Geometry: final body of the model. Coordinates: model frame, mm. Face numbers are marked on the shaded views. A direction names the side the tool comes from. Give positions to 0.01 mm unless a question says otherwise; leave off trailing zeros. Order: outer loops, then holes, each group sorted by start corner. A loop starts at its lowest first (then second) coordinate and runs counter-clockwise, first axis right, second up. Notation, with made-up numbers: (37.25, 64.5) - (67.25, 64.5) arc R34 ccw to (67.25, 96.5) - close; hole circle Ø9 at (71, 36.5). An arc over 180 degrees is marked (long way). Use one line per item in the form item = value.
from build123d import *

# Parameters (mm, degrees)
SKETCH1_W           = 39.99992
SKETCH1_H           = 19.99996
BOSS_EXTRUDE1_DEPTH = 9.0000074
BOSS_EXTRUDE2_DEPTH = 2.00000108
CHAMFER2_SIZE       = 1.00000054
SKETCH3_R           = 6.9999987
BOSS_EXTRUDE3_DEPTH = 1.00000054
SKETCH4_R           = 5.5000017
BOSS_EXTRUDE4_DEPTH = 1.00000054
SKETCH5_R           = 2.999994
CUT_EXTRUDE1_DEPTH  = 2.54
BOSS_EXTRUDE5_DEPTH = 1.999996
FILLET1_R           = 0.7500112
BOSS_EXTRUDE6_DEPTH = 0.50000027


with BuildPart() as part:
    # Sketch1 → Boss-Extrude1 (new body)
    with BuildSketch(Plane.XY):
        Rectangle(SKETCH1_W, SKETCH1_H)
    extrude(amount=BOSS_EXTRUDE1_DEPTH)

    # Sketch2 → Boss-Extrude2 (add)
    with BuildSketch(Plane.XY.offset(9.0000074)):
        with BuildLine():
            Line((14.99997, 9.99998), (-9.99998, 9.99998))
            ThreePointArc((-9.99998, 9.99998), (-19.99996, 0), (-9.99998, -9.99998))
            Line((-9.99998, -9.99998), (14.99997, -9.99998))
            Line((14.99997, -9.99998), (14.99997, 9.99998))
        make_face()
    extrude(amount=BOSS_EXTRUDE2_DEPTH)

    # Chamfer2
    chamfer2_edges = [part.edges().sort_by_distance(p)[0] for p in [
        (2.499995, -9.99998, 11.00000848),
        (-19.99996, 0, 11.00000848),
        (2.499995, 9.99998, 11.00000848),
        (14.99997, 0, 11.00000848),
    ]]
    chamfer(chamfer2_edges, length=CHAMFER2_SIZE)

    # Sketch3 → Boss-Extrude3 (add)
    with BuildSketch(Plane.XY.offset(11.00000848)):
        with Locations((-10.24995918, 0)):
            Circle(SKETCH3_R)
    extrude(amount=BOSS_EXTRUDE3_DEPTH)

    # Sketch4 → Boss-Extrude4 (add)
    with BuildSketch(Plane.XY.offset(12.00000902)):
        with Locations((-10.24995918, 0)):
            Circle(SKETCH4_R)
    extrude(amount=BOSS_EXTRUDE4_DEPTH)

    # Sketch5 → Cut-Extrude1 (cut)
    with BuildSketch(Plane.XY.offset(13.00000956)):
        with Locations((-10.24995918, 0)):
            Circle(SKETCH5_R)
    extrude(amount=-CUT_EXTRUDE1_DEPTH, mode=Mode.SUBTRACT)

    # Sketch6 → Boss-Extrude5 (add)
    with BuildSketch(Plane(origin=(0, 0, 0), x_dir=(-1, 0, 0), z_dir=(0, 0, -1))):
        with BuildLine():
            Line((27.027886, 8.99997946), (19.99996, 8.99997946))
            Line((19.99996, 8.99997946), (19.99996, -8.99997946))
            Line((19.99996, -8.99997946), (27.027886, -8.99997946))
            Line((27.027886, -8.99997946), (27.027886, -6.115627342))
            Line((27.027886, -6.115627342), (26.033157804, -6.115627342))
            ThreePointArc((26.033157804, -6.115627342), (22.40296035, -4.615626532), (26.033157804, -3.115625722))
            Line((26.033157804, -3.115625722), (27.027886, -3.115625722))
            Line((27.027886, -3.115625722), (27.027886, 3.115623182))
            Line((27.027886, 3.115623182), (26.033157804, 3.115623182))
            ThreePointArc((26.033157804, 3.115623182), (22.40296035, 4.615623992), (26.033157804, 6.115624802))
            Line((26.033157804, 6.115624802), (27.027886, 6.115624802))
            Line((27.027886, 6.115624802), (27.027886, 8.99997946))
        make_face()
    boss_extrude5 = extrude(amount=-BOSS_EXTRUDE5_DEPTH)

    # Fillet1
    fillet1_edges = [part.edges().sort_by_distance(p)[0] for p in [
        (-27.027886, -8.99997946, 0.999998),
        (-27.027886, 8.99997946, 0.999998),
    ]]
    fillet(fillet1_edges, radius=FILLET1_R)

    # Sketch7 → Boss-Extrude6 (add, symmetric)
    with BuildSketch(Plane(origin=(0, 0, 0), x_dir=(1, 0, 0), z_dir=(0, 1, 0))):
        Polygon((-27.027886, -1.999996), (-19.99996, -2.99999654), (-19.99996, -1.999996), align=None)
    boss_extrude6 = extrude(amount=BOSS_EXTRUDE6_DEPTH, both=True)

    # Mirror1: Boss-Extrude5, Boss-Extrude6 across plane
    add(boss_extrude5.mirror(Plane(origin=(0, 0, 0), x_dir=(0, 0, 1), z_dir=(1, 0, 0))))
    add(boss_extrude6.mirror(Plane(origin=(0, 0, 0), x_dir=(0, 0, 1), z_dir=(1, 0, 0))))


solid = part.part
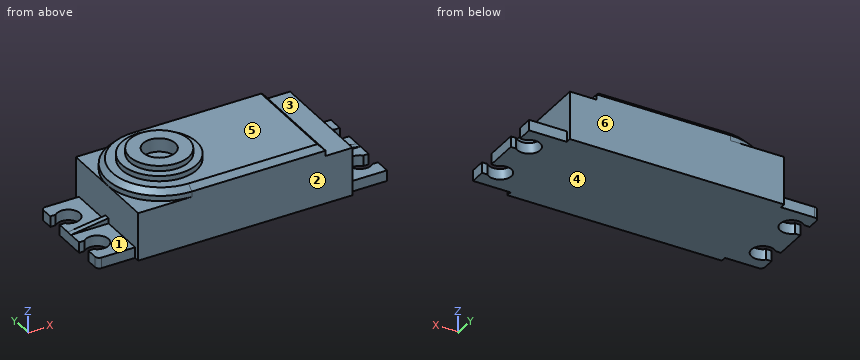
(1) Cut plane B-B on x = -0.5. Output: boundary loops of the cut face in (y, z), plus the area to 3 significant figures.
Computed values:
outline = (-10, 0) - (10, 0) - (10, 10) - (9, 11) - (-9, 11) - (-10, 10) - close
area = 219 mm²
(2) Ray query, line 1 along Y through (x, z) = (23, 1.25); line 2 along Z through (x, y) = (-12, 7.75); line 3 along X through (y, z) = (-9, 5). Return the intervals inside material, ascending.
Computed values:
line_1 = -9 to -6.09, -3.14 to 3.14, 6.09 to 9
line_2 = 0 to 11
line_3 = -20 to 20
(3) Reachability of the marked faces 1, 2 and 3 from +Z, -Z, +X, -X, +Y, -Y: full face, straight path, thin tool, end or side. Return the list, or none.
Computed values:
face_1 = +Z, -X, -Y
face_2 = +Z, -Z, +X, -X, -Y
face_3 = +Z, +X, +Y, -Y
(4) Pull-direction query (Z, two-part tool) for the marked faces 4, 5 and 6; classes: released by +Z, released by -Z, zero draft, split by the parting line, or undercut.
Computed values:
face_4 = released by -Z
face_5 = released by +Z
face_6 = zero draft
(5) Cut plane C-C on z = 6.5. Output: boundary loops of the cut face in (x, y), plus the area to 3 significant figures.
Computed values:
outline = (-20, -10) - (20, -10) - (20, 10) - (-20, 10) - close
area = 800 mm²
(6) Contact query for flat-ended pins moving along their axis: pin 1 Ø0.8 at (x, z) = (26.5, 1.5) entering from +Y; pin 2 Ø4 at (y, z) = (7.5, 7.5) entering from -X; pin 3 Ø7.5 at (x, y) = (-23, 6) entering from +Z. Output: stop coordinate, or through.
Computed values:
pin_1 = 9
pin_2 = -20
pin_3 = 9
